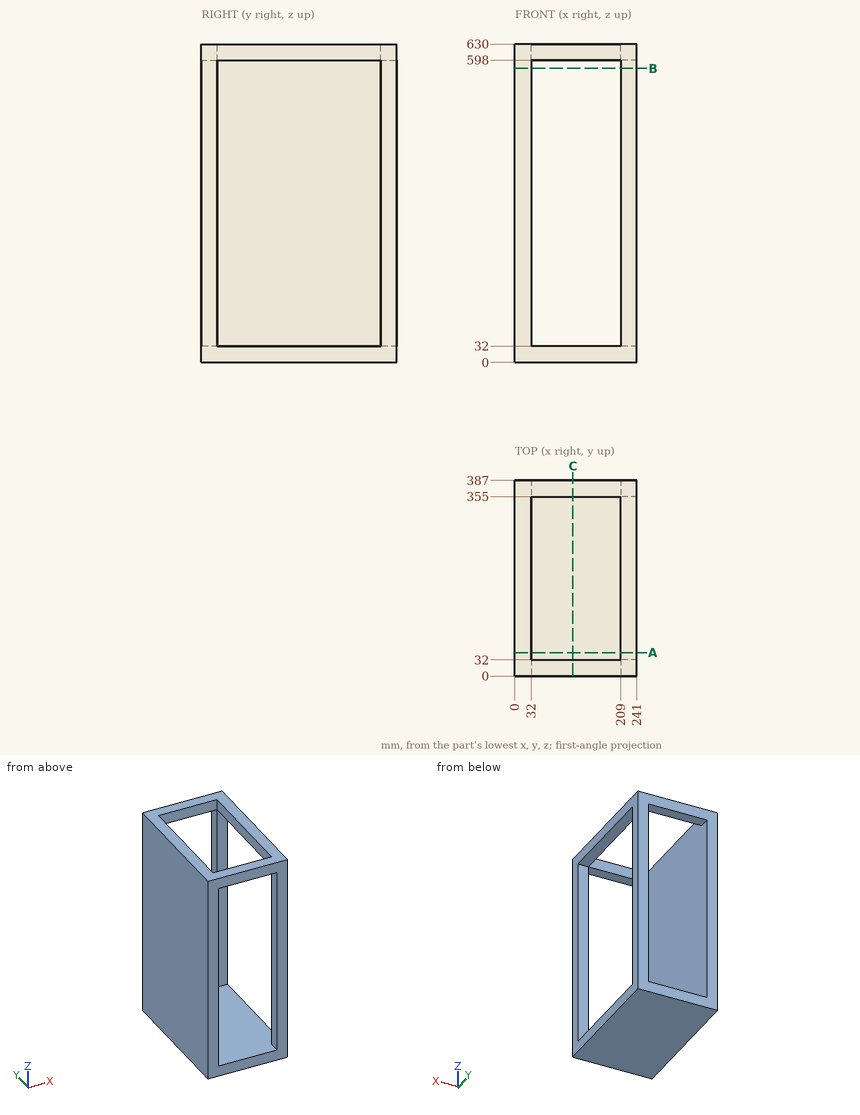
For this review, use the dimensioned drawing (mm, ordinates from the lowest corner) and the shaded views. Give positions to 0.01 mm unless a question says otherwise; leave off trailing zeros. Loops run counter-clockwise (first coordinate to the right, second up) from the corner with the lowest first, then second, coordinate; pieces in that order, holes last. Notation, with made-up numbers: (83.25, 29) -> (130.25, 29) arc R17 cw to (130.25, 62) -> close; hole circle Ø8 at (68.25, 5.25). An arc over 180 degrees is marked (long way). Use CSV: the item, a comma, the result in double quotes.
1. Consider section B-B, the plane z = 582. Write out the cut boundary in (x, y), then the cut area to 3 significant figures.
Result:
outline,"(0, 0) -> (32, 0) -> (32, 387) -> (0, 387) -> close; (209, 0) -> (241, 0) -> (241, 32) -> (209, 32) -> close; (209, 355) -> (241, 355) -> (241, 387) -> (209, 387) -> close"
area,"14,400 mm²"
2. To check wall thickness, follow probe 1 along X at (y, z) = (30.5, 188.5); probe 2 along Z at (x, y) = (114, 20.5); probe 3 along Y at (x, z) = (99, 600.5). State the ranges of each line that lie inside material, in increasing order. Write a range as from..to.
Result:
probe 1,"x = 0..32, 209..241"
probe 2,"z = 0..32, 598..630"
probe 3,"y = 0..32, 355..387"
3. Consider section C-C, the plane x = 114.5. Write out the cut boundary in (y, z).
Result:
outline,"(0, 0) -> (387, 0) -> (387, 32) -> (0, 32) -> close; (0, 598) -> (32, 598) -> (32, 630) -> (0, 630) -> close; (355, 598) -> (387, 598) -> (387, 630) -> (355, 630) -> close"
4. For P1, Ø12, axis at x = 109.5, y = 183.5, coming from the +Z side; P2, Ø8, axis at y = 202, z = 294.5, coming from the +X side, all flat-tipped, find the tip position at first contact; note any pin that passes through.
Result:
P1,"stops at z = 32"
P2,"stops at x = 32"
5. Consider section A-A, the plane y = 46. Write out the cut boundary in (x, z), then the cut area to 3 significant figures.
Result:
outline,"(0, 0) -> (241, 0) -> (241, 32) -> (32, 32) -> (32, 630) -> (0, 630) -> close; (209, 598) -> (241, 598) -> (241, 630) -> (209, 630) -> close"
area,"27,900 mm²"
